The listing builds one solid part. Answer for the finished solid, in the listing's coordinates (mm). Face numbers are marked on the shaded views. A direction names the side the tool comes from. Round coordinates to 2 decimals unless told otherwise and drop trailing zeros. Write each loop counter-clockwise with the first axis right and the second up, starting at its lowest first coordinate (ties: lowest second). Pieces come first, ordered by that corner, then holes.
from build123d import *

# Parameters (mm, degrees)
SKETCH1_R               = 2.5
BOSS_EXTRUDE1_DEPTH     = 6.35
SKETCH12_W              = 20
SKETCH12_H              = 6.35
BOSS_EXTRUDE2_DEPTH     = 6
FILLET2_R               = 3
SKETCH13_R              = 2.5
CUT_EXTRUDE9_DEPTH      = 1
CUT_EXTRUDE9_DEPTH_BACK = 7.35
FILLET1_R               = 3


with BuildPart() as part:
    # Sketch1 → Boss-Extrude1 (new body)
    with BuildSketch(Plane.XY):
        with BuildLine():
            Line((-37.5, -20), (11.5, -20))
            Line((11.5, -20), (11.5, -22))
            ThreePointArc((11.5, -22), (17.5, -28), (23.5, -22))
            Line((23.5, -22), (23.5, -20))
            Line((23.5, -20), (37.5, -20))
            Line((37.5, -20), (37.5, 20))
            Line((37.5, 20), (31.5, 20))
            Line((31.5, 20), (31.5, 21))
            ThreePointArc((31.5, 21), (25.5, 27), (19.5, 21))
            Line((19.5, 21), (19.5, 20))
            Line((19.5, 20), (-37.5, 20))
            Line((-37.5, 20), (-37.5, -20))
        make_face()
        with Locations((25.5, 21)):
            Circle(SKETCH1_R, mode=Mode.SUBTRACT)
        with Locations((17.5, -22)):
            Circle(SKETCH1_R, mode=Mode.SUBTRACT)
    extrude(amount=BOSS_EXTRUDE1_DEPTH)

    # Sketch12 → Boss-Extrude2 (add)
    with BuildSketch(Plane(origin=(0, 20, 0), x_dir=(1, 0, 0), z_dir=(0, 1, 0))):
        with Locations((0, -3.175)):
            Rectangle(SKETCH12_W, SKETCH12_H)
    extrude(amount=BOSS_EXTRUDE2_DEPTH)

    # Fillet2
    fillet2_edges = [part.edges().sort_by_distance(p)[0] for p in [
        (10, 20, 3.175),
        (-10, 20, 3.175),
    ]]
    fillet(fillet2_edges, radius=FILLET2_R)

    # Sketch13 → Cut-Extrude9 (cut, two sides)
    with BuildSketch(Plane.XY.offset(6.35)) as cut_extrude9_sk:
        with BuildLine():
            Line((-12.25, 20), (-37.5, 20))
            Line((-37.5, 20), (-37.5, -20))
            Line((-37.5, -20), (-12.25, -20))
            ThreePointArc((-12.25, -20), (-19.075859236, -18.799139494), (-25.082027993, -15.34076457))
            Line((-25.082027993, -15.34076457), (-29.549349609, -18.20790773))
            ThreePointArc((-29.549349609, -18.20790773), (-36.45790773, -16.700650391), (-34.950650391, -9.79209227))
            Line((-34.950650391, -9.79209227), (-30.909610133, -7.198538025))
            ThreePointArc((-30.909610133, -7.198538025), (-32.25, 0), (-30.909610133, 7.198538025))
            Line((-30.909610133, 7.198538025), (-34.950650391, 9.79209227))
            ThreePointArc((-34.950650391, 9.79209227), (-36.45790773, 16.700650391), (-29.549349609, 18.20790773))
            Line((-29.549349609, 18.20790773), (-25.082027993, 15.34076457))
            ThreePointArc((-25.082027993, 15.34076457), (-19.075859236, 18.799139494), (-12.25, 20))
        make_face()
        with Locations((-32.25, 14)):
            Circle(SKETCH13_R)
        with Locations((-32.25, -14)):
            Circle(SKETCH13_R)
    extrude(amount=CUT_EXTRUDE9_DEPTH, mode=Mode.SUBTRACT)
    extrude(cut_extrude9_sk.sketch, amount=-CUT_EXTRUDE9_DEPTH_BACK, mode=Mode.SUBTRACT)

    # Fillet1
    fillet1_edges = [part.edges().sort_by_distance(p)[0] for p in [
        (11.5, -20, 3.175),
        (23.5, -20, 3.175),
        (31.5, 20, 3.175),
        (19.5, 20, 3.175),
        (-25.082027993, -15.34076457, 3.175),
        (-25.082027993, 15.34076457, 3.175),
        (-30.909610133, -7.198538025, 3.175),
        (-30.909610133, 7.198538025, 3.175),
    ]]
    fillet(fillet1_edges, radius=FILLET1_R)


solid = part.part
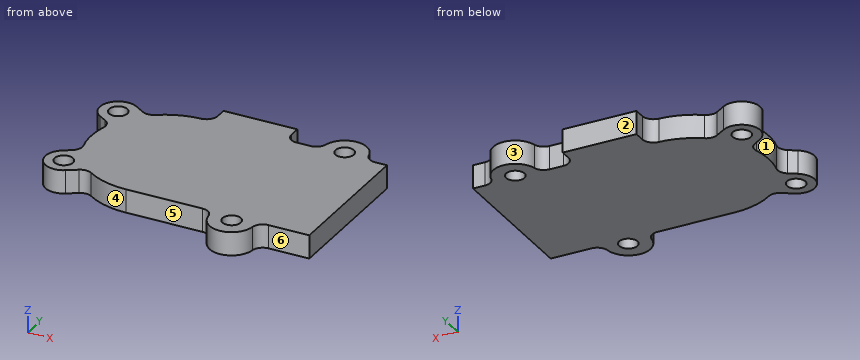
1. Straight lines are drawn through the part: line 1 along Y through (x, z) = (-20.5, 3.5); line 2 along Y through (x, z) = (26, 1); line 3 along X through (y, z) = (6, 0.5). For each, find the intervals that lie inside material, in ascending order.
Geometry says:
line 1: y = -18.22 to 18.22
line 2: y = -20.03 to 18.55, 23.45 to 26.98
line 3: x = -31.48 to 37.5
2. A tool of negligible diameter and unlimited length cuts with its end or side. For the marked faces 4, 5 and 6, from which of +Z, -Z, +X, -X, +Y, -Y can it reach the whole face along a straight path? Write none if from no direction.
Geometry says:
face 4: +Z, -Z, -Y
face 5: +Z, -Z, -X, -Y
face 6: +Z, -Z, +X, -Y
3. Section B-B on z = 3.5 is taken. Give the number of separate pieces and of enclosed holes in the cut face, plus the area to 3 significant figures.
Geometry says:
separate pieces: 1
enclosed holes: 4
area: 2,990 mm2
4. For a pull along X with two mould halves and no side action, classify the marked faces 1, 2 and 3 as released by +X, released by -X, zero draft, split by the parting line, or undercut.
Geometry says:
face 1: released by -X
face 2: zero draft
face 3: undercut
5. Section A-A on y = 14 is taken. Determine the outline of the cut face in (x, z).
Geometry says:
outline: (-37.25, 0) - (-34.75, 0) - (-34.75, 6.35) - (-37.25, 6.35) - close; (-29.75, 0) - (37.5, 0) - (37.5, 6.35) - (-29.75, 6.35) - close
6. Given pin 1 (4 mm diameter, centred on x = 13, y = 2, fed in from -Z); pin 2 (1.5 mm diameter, centred on y = 24.5, z = 2, fed in from +X); pin 3 (1 mm diameter, centred on y = 0, z = 1, fed in from -X); pin 4 (3 mm diameter, centred on x = 1.5, z = 4.5, fed in from -Y), each flat-ended and moving along its own axis, determine where each tip first touches the part or whether it passes through.
Geometry says:
pin 1: stops at z = 0
pin 2: stops at x = 30.83
pin 3: stops at x = -32.25
pin 4: stops at y = -20
7. Section C-C on x = 4.5 is taken. Determine the outline of the cut face in (y, z), plus the area to 3 significant figures.
Geometry says:
outline: (-20, 0) - (26, 0) - (26, 6.35) - (-20, 6.35) - close
area: 292 mm2
